Geometry: final body of the model. Coordinates: model frame, mm. Round coordinates to 2 decimals unless told otherwise and drop trailing zeros. Loops run counter-clockwise (first coordinate to the right, second up) from the corner with the lowest first, then second, coordinate; pieces in that order, holes last. Notation, with made-up numbers: (-10, 32.5) - (3, 32.5) arc R12 cw to (3, 41.5) - close; hole circle Ø8 at (-38.75, 5). An arc over 180 degrees is marked (long way). Write item = value, one per line. Start each with the question number.
Item 1: Line query: line 1 (Z direction, x = -6.5, y = 33.7); line 2 (Z direction, x = -6, y = 13); line 3 (X direction, y = 17, z = 30). Output: solid intervals per line, ascending. Write a range as from..to.
Item 2: Section B-B (z = 30). Return loops of the section in (x, y), plus the area to 3 significant figures.
Item 3: Section A-A (x = -6.5). Return loops of the section in (y, z).
Item 4: Draft query along X for faces 1 (the flat face through (-2, 33, 35)), 2 (the flat face through (-1, -26, 23)), 3 (the flat face through (-87.5, 4, 30)), 4 (the cylindrical face through (-8.88, 33.51, 40.74)). Return one class per face: pulls with the +X half, pulls with the -X half, needs draft (parallel to the pull), parting line crosses it, or undercut.
from build123d import *

# Parameters (mm, degrees)
ESQUISSE1_W          = 175
ESQUISSE1_H          = 60
EXTRUSION1_DEPTH     = 60
PER_AGE1_D           = 11.5
PER_AGE1_CBORE_D     = 22
PER_AGE1_CBORE_DEPTH = 1


with BuildPart() as part:
    # Esquisse1 → Extrusion1 (new body)
    with BuildSketch(Plane.XY):
        with Locations((0, 4)):
            Rectangle(ESQUISSE1_W, ESQUISSE1_H)
    extrude(amount=EXTRUSION1_DEPTH)

    # Perçage1 (through all)
    with Locations(Plane(origin=(-6.5, 34, 30), x_dir=(1, 0, 0), z_dir=(0, 1, 0))):
        with Locations((0, 0)):
            CounterBoreHole(PER_AGE1_D / 2, PER_AGE1_CBORE_D / 2, PER_AGE1_CBORE_DEPTH)


solid = part.part
Taken from the geometry:
q1.line_1 = 0..19, 41..60
q1.line_2 = 0..24.27, 35.73..60
q1.line_3 = -87.5..-12.25, -0.75..87.5
q2.outline = (-87.5, -26) - (-12.25, -26) - (-12.25, 33) - (-17.5, 33) - (-17.5, 34) - (-87.5, 34) - close; (-0.75, -26) - (87.5, -26) - (87.5, 34) - (4.5, 34) - (4.5, 33) - (-0.75, 33) - close
q2.area = 9,800 mm^2
q3.outline = (-26, 0) - (34, 0) - (34, 19) - (33, 19) - (33, 24.25) - (-26, 24.25) - close; (-26, 35.75) - (33, 35.75) - (33, 41) - (34, 41) - (34, 60) - (-26, 60) - close
q4.face_1 = undercut
q4.face_2 = needs draft
q4.face_3 = pulls with the -X half
q4.face_4 = undercut
